```python
from build123d import *

# Parameters (mm, degrees)
F1_DEPTH      = 10
F4_ANGLE      = -30
F6_COUNT      = 6
F0_R          = 15
F7_DEPTH      = 13.2
F7_DEPTH_BACK = 3.5


with BuildPart() as f1:
    # F0 (on Top) → F1 (new body)
    with BuildSketch(Plane.XY):
        with BuildLine():
            Line((36.5413986146, 63.2915589802), (15, 25.9807621135))
            ThreePointArc((15, 25.9807621135), (21.2132034356, 21.2132034356), (25.9807621135, 15))
            Line((25.9807621135, 15), (86.6025403784, 50))
            ThreePointArc((86.6025403784, 50), (70.7106781187, 70.7106781187), (50, 86.6025403784))
            Line((50, 86.6025403784), (36.5413986146, 63.2915589802))
        make_face()
        with BuildLine():
            ThreePointArc((25.9807621135, 15), (21.2132034356, 21.2132034356), (15, 25.9807621135))
            Line((15, 25.9807621135), (10.982790001, 19.0227502905))
            ThreePointArc((10.982790001, 19.0227502905), (15.5320105721, 15.5320105721), (19.0227502905, 10.982790001))
            Line((19.0227502905, 10.982790001), (25.9807621135, 15))
        make_face()
    extrude(amount=F1_DEPTH)


with BuildPart() as f1_1:
    # F4: moved
    add(f1.part.rotate(Axis((41.835274435, 42.0708136254, 5), (-0.709996604, -0.7042050996, 0)), F4_ANGLE))


with BuildPart() as f6_1:
    # F6: instance of F1
    add(f1_1.part.rotate(Axis((0, 0, -5.4106004536), (0, 0, -1)), 1 * 360 / F6_COUNT))


with BuildPart() as f6_2:
    # F6: instance of F1
    add(f1_1.part.rotate(Axis((0, 0, -5.4106004536), (0, 0, -1)), 2 * 360 / F6_COUNT))


with BuildPart() as f6_3:
    # F6: instance of F1
    add(f1_1.part.rotate(Axis((0, 0, -5.4106004536), (0, 0, -1)), 3 * 360 / F6_COUNT))


with BuildPart() as f6_4:
    # F6: instance of F1
    add(f1_1.part.rotate(Axis((0, 0, -5.4106004536), (0, 0, -1)), 4 * 360 / F6_COUNT))


with BuildPart() as f6_5:
    # F6: instance of F1
    add(f1_1.part.rotate(Axis((0, 0, -5.4106004536), (0, 0, -1)), 5 * 360 / F6_COUNT))


with BuildPart() as f1_2:
    add(f1_1.part)

    add(f6_1.part)  # F7 merges F6_1

    add(f6_2.part)  # F7 merges F6_2

    add(f6_3.part)  # F7 merges F6_3

    add(f6_4.part)  # F7 merges F6_4

    add(f6_5.part)  # F7 merges F6_5
    # F0 (on Top) → F7 (join, two sides)
    with BuildSketch(Plane.XY) as f7_sk:
        with BuildLine():
            ThreePointArc((25.9807621135, 15), (21.2132034356, 21.2132034356), (15, 25.9807621135))
            Line((15, 25.9807621135), (10.982790001, 19.0227502905))
            ThreePointArc((10.982790001, 19.0227502905), (15.5320105721, 15.5320105721), (19.0227502905, 10.982790001))
            Line((19.0227502905, 10.982790001), (25.9807621135, 15))
        make_face()
        with BuildLine():
            Line((10.982790001, 19.0227502905), (15, 25.9807621135))
            ThreePointArc((15, 25.9807621135), (-25.9807621135, -15), (30, 0))
            ThreePointArc((30, 0), (28.9777747887, 7.7645713531), (25.9807621135, 15))
            Line((25.9807621135, 15), (19.0227502905, 10.982790001))
            ThreePointArc((19.0227502905, 10.982790001), (15.5320105721, 15.5320105721), (10.982790001, 19.0227502905))
        make_face()
        Circle(F0_R, mode=Mode.SUBTRACT)
    extrude(amount=F7_DEPTH)
    extrude(f7_sk.sketch, amount=-F7_DEPTH_BACK)


solid = f1_2.part
```
For this review, take the finished solid that the model builds, in its own axes (mm). A direction names the side the tool comes from. Round coordinates to 2 decimals unless told otherwise and drop trailing zeros. One line per question, with ' | ' between items. Start each with the question number.
1) For pin 1 Ø3 at (y, z) = (39, 10) entering from -X; pin 2 Ø2 at (x, z) = (64, 16.5) entering from +Y; pin 3 Ø5 at (y, z) = (44.5, 13.5) entering from -X, all flat-tipped, find the tip position at first contact; note any pin that passes through.
2) Mouldability with a two-part tool opening along Y and no side actions: class faces 1 (the flat face through (-14, -6, 13.2)), 2 (the cylindrical face through (-25.609, 96.665, 4.756)), 3 (the cylindrical face through (96.52, -26.15, 4.76)) as +Y half, -Y half, draft (parallel to the pull), parting line (faces both ways), or undercut.
3) Add section A-A (z = -8). Count the separate pieces of the cut face and the enclosed holes in it, and give its area (3 significant figures).
4) Machinability: for faces 4 (the flat face through (-21.801, 68.595, 1.068)), 5 (the flat face through (48.5, 53.18, 1.07)), 6 (the flat face through (-70.306, 15.417, 1.068)), 7 (the flat face through (52.284, 49.392, 9.527)), which of the approach directions +Z, -Z, +X, -X, +Y, -Y give a long, thin tool a straight path to every point of the face, cutting with its end or side? Answer none if there is none.
5) Wall thickness on line 1 along Y through (x, z) = (0, -1); line 2 along X through (y, z) = (-75.5, 11); line 3 along Y through (x, z) = (-37, 2): over which ranges is each line inside the solid? List them lowest first.
Reported:
1) pin 1: stops at x = -22.61 | pin 2: stops at y = 76.95 | pin 3: stops at x = -24.71
2) face 1: undercut | face 2: +Y half | face 3: -Y half
3) separate pieces: 6 | enclosed holes: 0 | area: 1,020 mm²
4) face 4: -Z | face 5: -Z, +Y | face 6: -Z, -X | face 7: +Z, +X
5) line 1: y = -30 to -15, 15 to 30 | line 2: x = -65.3 to -46.58, 20.73 to 41.41 | line 3: y = -44.04 to -21.34, 4.67 to 21.38
